For this review, use the dimensioned drawing (mm, ordinates from the lowest corner) and the shaded views. A direction names the side the tool comes from. Coordinates: 2 decimals unless noted, no trailing zeros. Write each loop counter-clockwise with the first axis right and the second up, starting at its lowest first coordinate (ties: lowest second). Pieces come first, ordered by that corner, then holes.
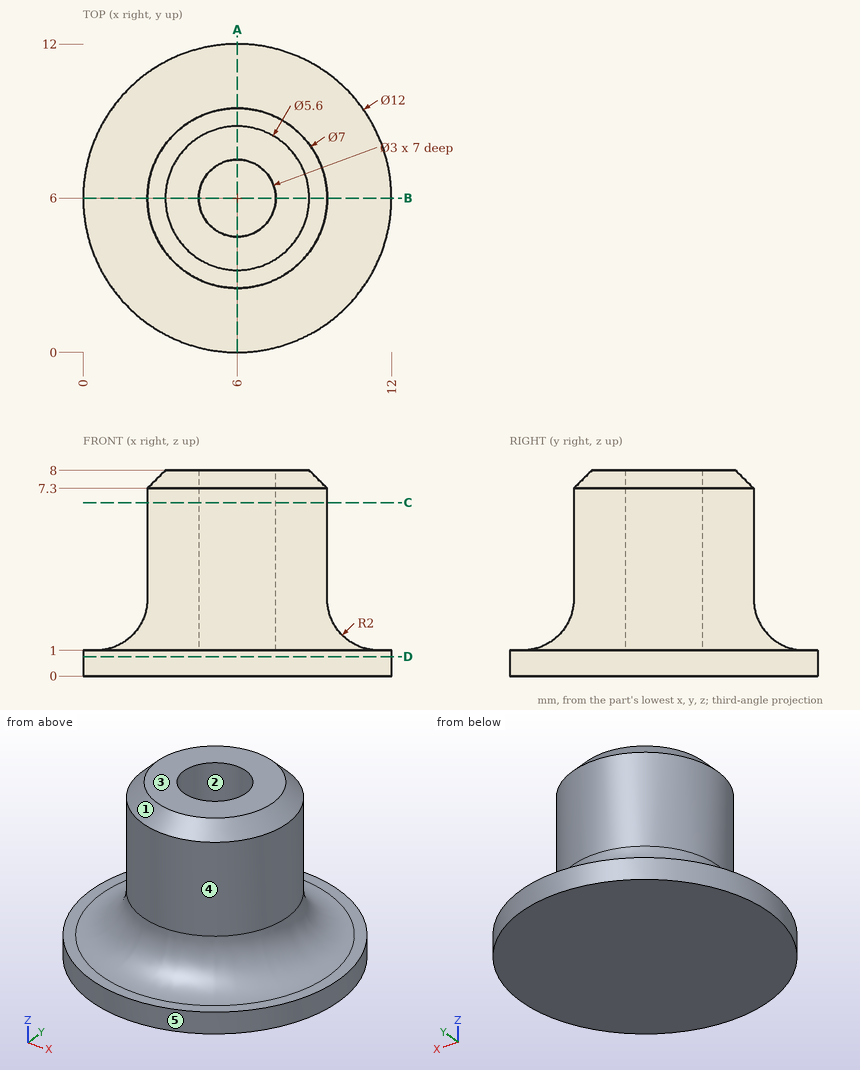
Item 1: Machinability: for the marked faces 4 and 5, which of the approach directions +Z, -Z, +X, -X, +Y, -Y give a long, thin tool a straight path to every point of the face, cutting with its end or side? Answer none if there is none.
Solved:
face 4: +Z
face 5: +Z, -Z
Item 2: For pin 1 (2.5 mm diameter, centred on x = 6, y = 6, fed in from +Z); pin 2 (1.5 mm diameter, centred on x = 7.5, z = 3.5, fed in from +Y), all flat-tipped, find the tip position at first contact; note any pin that passes through.
Solved:
pin 1: stops at z = 1
pin 2: stops at y = 9.42
Item 3: Take a section at D-D, the plane z = 0.75. Write out the cut boundary in (x, y).
Solved:
outline: circle Ø12 at (6, 6)
Item 4: Take a section at C-C, the plane z = 6.75. Write out the cut boundary in (x, y), plus the area to 3 significant figures.
Solved:
outline: circle Ø7 at (6, 6); hole circle Ø3 at (6, 6)
area: 31.4 mm2
Item 5: Mouldability with a two-part tool opening along X and no side actions: class the marked faces 1, 2 and 3 as pulls with the +X half, pulls with the -X half, needs draft (parallel to the pull), parting line crosses it, or undercut.
Solved:
face 1: parting line crosses it
face 2: undercut
face 3: needs draft
Item 6: Take a section at A-A, the plane x = 6. Write out the cut boundary in (y, z).
Solved:
outline: (0, 0) - (12, 0) - (12, 1) - (11.5, 1) arc R2 cw to (9.5, 3) - (9.5, 7.3) - (8.8, 8) - (7.5, 8) - (7.5, 1) - (4.5, 1) - (4.5, 8) - (3.2, 8) - (2.5, 7.3) - (2.5, 3) arc R2 cw to (0.5, 1) - (0, 1) - close
Item 7: To check wall thickness, follow line 1 along Y through (x, z) = (6, 6.5); line 2 along X through (y, z) = (7, 6.75). State the ranges of each line that lie inside material, in increasing order.
Solved:
line 1: y = 2.5 to 4.5, 7.5 to 9.5
line 2: x = 2.65 to 4.88, 7.12 to 9.35
